The listing builds one solid part. Answer for the finished solid, in the listing's coordinates (mm). A direction names the side the tool comes from. Coordinates: 2 decimals unless noted, no trailing zeros. Order: outer loops, then holes, each group sorted by start corner. A loop starts at its lowest first (then second) coordinate and runs counter-clockwise, first axis right, second up.
```python
from build123d import *

# Parameters (mm, degrees)
F0_W     = 70.4235509038
F0_H     = 96.9706401229
F1_DEPTH = 25.4
F2_W     = 153.4230113029
F2_H     = 40.9747579411
F2_W_2   = 70.4235509038
F2_H_2   = 25.4
F3_DEPTH = 25.4
F4_W     = 42.5563007593
F4_H     = 61.9181990623
F5_DEPTH = 25.4


with BuildPart() as f1:
    # F0 (on Front) → F1 (new body)
    with BuildSketch(Plane.XZ):
        Rectangle(F0_W, F0_H)
    extrude(amount=F1_DEPTH)

    # F2 (on face) → F3 (join)
    with BuildSketch(Plane.XY.offset(48.4853200614)):
        with Locations((0, -12.7)):
            Rectangle(F2_W, F2_H)
        with Locations((0, -12.7)):
            Rectangle(F2_W_2, F2_H_2, mode=Mode.SUBTRACT)
        with Locations((0, -12.7)):
            Rectangle(F2_W_2, F2_H_2)
    extrude(amount=F3_DEPTH)

    # F4 (on face) → F5 (cut)
    with BuildSketch(Plane.XZ.offset(25.4)):
        Rectangle(F4_W, F4_H)
    extrude(amount=-F5_DEPTH, mode=Mode.SUBTRACT)


solid = f1.part
```
1) A cutting plane is placed at C-C, the plane y = -10. Write down the section's boundary in (x, z).
2) The mould has two halves that part along Z. Classify faces 1 (the flat face through (0, -13, -48.485)), 2 (the flat face through (-21.278, -13, 0)), 3 (the flat face through (0, -13, -30.959)), 4 (the flat face through (-35.212, -13, -1)): released by +Z, released by -Z, zero draft, split by the parting line, or undercut.
3) A cutting plane is placed at D-D, the plane x = 26. Write down the section's boundary in (y, z).
4) Each of these flat-tipped pins is pushed along its axis until it touches: P1, Ø21, axis at x = -5, z = -20.5, coming from the +Y side; P2, Ø12.5, axis at y = -17, z = 0, coming from the +X side; P3, Ø8, axis at y = 3.5, z = 36, coming from the -X side; P4, Ø21, axis at x = 2.5, z = -6, coming from the -Y side. Where does it stop, or does it pass through?
5) For faces 5 (the flat face through (35.212, -13, -1)), 6 (the flat face through (-24, -25.4, 1)), 7 (the flat face through (0, -13, 30.959)), determine the directions among +Z, -Z, +X, -X, +Y, -Y from which every point of the face is accessible in a straight line to the end or side of a thin tool.
6) A cutting plane is placed at B-B, the plane z = -7. Write down the section's boundary in (x, y), plus the area to 3 significant figures.
7) Straight lines are drawn through the part: probe 1 along X at (y, z) = (-14.5, -14.5); probe 2 along Z at (x, y) = (-5, -24); probe 3 along X at (y, z) = (-4, -40.5). For each, find the intervals that lie inside material, in ascending order.
8) A cutting plane is placed at A-A, the plane x = -8. Write down the section's boundary in (y, z).
Working result:
1. outline: (-76.71, 48.49) - (-35.21, 48.49) - (-35.21, -48.49) - (35.21, -48.49) - (35.21, 48.49) - (76.71, 48.49) - (76.71, 73.89) - (-76.71, 73.89) - close; hole (-21.28, -30.96) - (21.28, -30.96) - (21.28, 30.96) - (-21.28, 30.96) - close
2. face 1: released by -Z
2. face 2: undercut
2. face 3: undercut
2. face 4: zero draft
3. outline: (-33.19, 48.49) - (-25.4, 48.49) - (-25.4, -48.49) - (0, -48.49) - (0, 48.49) - (7.79, 48.49) - (7.79, 73.89) - (-33.19, 73.89) - close
4. P1: stops at y = 0
4. P2: stops at x = 35.21
4. P3: stops at x = -35.21
4. P4: passes through
5. face 5: -Z, +X, +Y, -Y
5. face 6: -Z, +X, -X, -Y
5. face 7: +Y, -Y
6. outline: (-35.21, -25.4) - (-21.28, -25.4) - (-21.28, 0) - (-35.21, 0) - close; (21.28, -25.4) - (35.21, -25.4) - (35.21, 0) - (21.28, 0) - close
6. area: 708 mm2
7. probe 1: x = -35.21 to -21.28, 21.28 to 35.21
7. probe 2: z = -48.49 to -30.96, 30.96 to 73.89
7. probe 3: x = -35.21 to 35.21
8. outline: (-33.19, 48.49) - (-25.4, 48.49) - (-25.4, 30.96) - (0, 30.96) - (0, 48.49) - (7.79, 48.49) - (7.79, 73.89) - (-33.19, 73.89) - close; (-25.4, -48.49) - (0, -48.49) - (0, -30.96) - (-25.4, -30.96) - close
